Geometry: final body of the model. Coordinates: model frame, mm. A direction names the side the tool comes from. Give positions to 0.01 mm unless a question says otherwise; leave off trailing zeros. Loops run counter-clockwise (first coordinate to the right, second up) from the corner with the lowest first, then second, coordinate; pieces in that order, holes last. Notation, with made-up numbers: (-38, -5.5) -> (-18, -5.5) arc R13 cw to (-18, 15.5) -> close; hole circle Ø6 at (88, -38.5). An arc over 180 degrees is marked (long way). Answer in a Markdown table with one row per item. Add a question column.
1) Access query for faces 1 (the cylindrical face through (-113.36, 142.48, 6.34)), 2 (the flat face through (72.745, 132.247, 10.647)), 3 (the flat face through (80, 65, 6)). Directions: +Z, -Z, +X, -X, +Y, -Y. A direction counts if a zero-diameter tool reaches every point of the face in a straight line with its end or side. Return the directions, or none.
2) Draft query along Y for faces 4 (the cylindrical face through (84, 251, 16)), 5 (the flat face through (-74.9, 66.2, 17.6)), 6 (the conical face through (-74.64, 25.81, 17.57)). Return one class per face: +Y half, -Y half, draft (parallel to the pull), parting line (faces both ways), or undercut.
3) Section query B-B (z = 17.75). Give the number of separate pieces and of enclosed holes in the cut face, plus the area to 3 significant figures.
4) Line query: line 1 (X direction, y = 212.5, z = 3.5); line 2 (X direction, y = 254, z = 18); line 3 (X direction, y = 47.5, z = 1.75). Output: solid intervals per line, ascending. Write a range as from..to.
5) Section query A-A (y = 81). Return the cut outline in (x, z).
6) First-contact query: P1, Ø8, axis at x = -88, z = 14.5, coming from the -Y side; P2, Ø1.2, axis at y = 61, z = 5.5, coming from the +X side; P3, Ø1, axis at y = 140.5, z = 19.5, coming from the -X side. Flat tips, straight axial feed; report the tip coordinate or a pass-through.
```python
from build123d import *

# Parameters (mm, degrees)
RESSALTO_EXTRUS_O1_DEPTH = 22.5
CHANFRO1_SIZE            = 10
CORTE_EXTRUS_O1_REACH    = 305.531
ESBO_O3_W                = 1139.230904301
ESBO_O3_H                = 709.798033895
CORTE_EXTRUS_O5_DEPTH    = 1.5
ESBO_O5_R                = 3
CORTE_EXTRUS_O6_DEPTH    = 304.423796035
CORTE_EXTRUS_O8_DEPTH    = 10


with BuildPart() as part:
    # Esboço1 → Ressalto-extrusão1 (new, symmetric)
    with BuildSketch(Plane.XY):
        with BuildLine():
            Line((-55.336923418, 0), (55.336923418, 0))
            ThreePointArc((55.336923418, 0), (59.563106036, 0.93692213), (62.99736785, 3.572123903))
            Line((62.99736785, 3.572123903), (77.660444431, 21.046898098))
            ThreePointArc((77.660444431, 21.046898098), (79.396926208, 24.054572761), (80, 27.474774195))
            Line((80, 27.474774195), (80, 103.835071852))
            ThreePointArc((80, 103.835071852), (81.685949179, 111.43989715), (86.427876097, 117.619696626))
            Line((86.427876097, 117.619696626), (108.572123903, 136.200926793))
            ThreePointArc((108.572123903, 136.200926793), (113.314050821, 142.380726268), (115, 149.985551567))
            Line((115, 149.985551567), (115, 249.022509221))
            ThreePointArc((115, 249.022509221), (114.06307787, 253.248691838), (111.427876097, 256.682953652))
            Line((111.427876097, 256.682953652), (86.427876097, 277.660444431))
            ThreePointArc((86.427876097, 277.660444431), (83.420201433, 279.396926208), (80, 280))
            Line((80, 280), (-80, 280))
            ThreePointArc((-80, 280), (-83.420201433, 279.396926208), (-86.427876097, 277.660444431))
            Line((-86.427876097, 277.660444431), (-111.427876097, 256.682953652))
            ThreePointArc((-111.427876097, 256.682953652), (-114.06307787, 253.248691838), (-115, 249.022509221))
            Line((-115, 249.022509221), (-115, 149.985551567))
            ThreePointArc((-115, 149.985551567), (-113.314050821, 142.380726268), (-108.572123903, 136.200926793))
            Line((-108.572123903, 136.200926793), (-86.427876097, 117.619696626))
            ThreePointArc((-86.427876097, 117.619696626), (-81.685949179, 111.43989715), (-80, 103.835071852))
            Line((-80, 103.835071852), (-80, 27.474774195))
            ThreePointArc((-80, 27.474774195), (-79.396926208, 24.054572761), (-77.660444431, 21.046898098))
            Line((-77.660444431, 21.046898098), (-62.99736785, 3.572123903))
            ThreePointArc((-62.99736785, 3.572123903), (-59.563106036, 0.93692213), (-55.336923418, 0))
        make_face()
        Polygon((-90, 146.725210262), (-90, 236.228675506), (-61.670438633, 260), (61.670438633, 260), (90, 236.228675506), (90, 146.725210262), (55, 117.356723171), (55, 28.676328085), (47.719696304, 20), (-47.719696304, 20), (-55, 28.676328085), (-55, 117.356723171), align=None, mode=Mode.SUBTRACT)
    extrude(amount=RESSALTO_EXTRUS_O1_DEPTH, both=True)

    # Chanfro1
    chanfro1_edges = [part.edges().sort_by_distance(p)[0] for p in [
        (-70.32890614, 12.309511, 22.5),
        (-59.563106036, 0.93692213, 22.5),
        (0, 0, 22.5),
        (59.563106036, 0.93692213, 22.5),
        (70.32890614, 12.309511, 22.5),
        (79.396926208, 24.054572761, 22.5),
        (80, 65.654923023, 22.5),
        (81.685949179, 111.43989715, 22.5),
        (97.5, 126.910311709, 22.5),
        (113.314050821, 142.380726268, 22.5),
        (115, 199.504030394, 22.5),
        (114.06307787, 253.248691838, 22.5),
        (98.927876097, 267.171699041, 22.5),
        (98.927876097, 267.171699041, -22.5),
        (114.06307787, 253.248691838, -22.5),
        (115, 199.504030394, -22.5),
        (113.314050821, 142.380726268, -22.5),
        (97.5, 126.910311709, -22.5),
        (81.685949179, 111.43989715, -22.5),
        (80, 65.654923023, -22.5),
        (79.396926208, 24.054572761, -22.5),
        (70.32890614, 12.309511, -22.5),
        (59.563106036, 0.93692213, -22.5),
        (0, 0, -22.5),
        (-59.563106036, 0.93692213, -22.5),
        (-70.32890614, 12.309511, -22.5),
        (-79.396926208, 24.054572761, -22.5),
        (-80, 65.654923023, -22.5),
        (-81.685949179, 111.43989715, -22.5),
        (-97.5, 126.910311709, -22.5),
        (-113.314050821, 142.380726268, -22.5),
        (-115, 199.504030394, -22.5),
        (-114.06307787, 253.248691838, -22.5),
        (-98.927876097, 267.171699041, -22.5),
        (-83.420201433, 279.396926208, -22.5),
        (0, 280, -22.5),
        (83.420201433, 279.396926208, -22.5),
        (83.420201433, 279.396926208, 22.5),
        (0, 280, 22.5),
        (-83.420201433, 279.396926208, 22.5),
        (-98.927876097, 267.171699041, 22.5),
        (-114.06307787, 253.248691838, 22.5),
        (-115, 199.504030394, 22.5),
        (-113.314050821, 142.380726268, 22.5),
        (-97.5, 126.910311709, 22.5),
        (-81.685949179, 111.43989715, 22.5),
        (-80, 65.654923023, 22.5),
        (-79.396926208, 24.054572761, 22.5),
    ]]
    chamfer(chanfro1_edges, length=CHANFRO1_SIZE - 0.0001)  # a hair under: the kernel refuses the full size

    # Esboço3 → Corte-extrusão1 (cut, up to next)
    with BuildSketch(Plane.XY, mode=Mode.PRIVATE) as corte_extrus_o1_sk1:
        with Locations((-153.157436203, 152.53565808)):
            Rectangle(ESBO_O3_W, ESBO_O3_H)
    corte_extrus_o1_tool1 = extrude(corte_extrus_o1_sk1.sketch, amount=-CORTE_EXTRUS_O1_REACH, mode=Mode.PRIVATE) & part.part
    add(corte_extrus_o1_tool1.solids().sort_by_distance((-153.157436, 152.535658, 0))[0], mode=Mode.SUBTRACT)

    # Esboço4 → Corte-extrusão5 (cut)
    with BuildSketch(Plane.XY.offset(22.5)):
        Polygon((-69, 27.838744429), (-54.87061576, 11), (54.87061576, 11), (69, 27.838744429), (69, 117.355452403), (104, 146.723939495), (104, 248.556201562), (79.636029766, 269), (-79.636029766, 269), (-104, 248.556201562), (-104, 146.723939495), (-69, 117.355452403), align=None)
        Polygon((-90, 146.725210262), (-90, 236.228675506), (-61.670438633, 260), (61.670438633, 260), (90, 236.228675506), (90, 146.725210262), (55, 117.356723171), (55, 28.676328085), (47.719696304, 20), (-47.719696304, 20), (-55, 28.676328085), (-55, 117.356723171), align=None, mode=Mode.SUBTRACT)
    extrude(amount=-CORTE_EXTRUS_O5_DEPTH, mode=Mode.SUBTRACT)

    # Esboço5 → Corte-extrusão6 (cut, through all)
    with BuildSketch(Plane.XY.offset(21)):
        with Locations((-97, 244)):
            Circle(ESBO_O5_R)
        with Locations((-62, 60.396230411)):
            Circle(ESBO_O5_R)
        with Locations((-84, 254)):
            Circle(ESBO_O5_R)
        with Locations((-55, 21)):
            Circle(ESBO_O5_R)
        with Locations(Location((55, 21, 0), (0, 0, 180))):
            Circle(ESBO_O5_R)
        with Locations(Location((84, 254, 0), (0, 0, 180))):
            Circle(ESBO_O5_R)
        with Locations(Location((62, 60.396230411, 0), (0, 0, 180))):
            Circle(ESBO_O5_R)
        with Locations(Location((97, 244, 0), (0, 0, 180))):
            Circle(ESBO_O5_R)
    extrude(amount=-CORTE_EXTRUS_O6_DEPTH, mode=Mode.SUBTRACT)

    # Esboço7 → Corte-extrusão8 (cut)
    with BuildSketch(Plane(origin=(0, 0, 0), x_dir=(-1, 0, 0), z_dir=(0, 0, -1))):
        Polygon((83.862394336, 258.039108567), (80.43322654, 255.900384282), (80.570832205, 251.861275715), (84.137605664, 249.960891433), (87.56677346, 252.099615718), (87.429167795, 256.138724285), align=None)
        Polygon((-96.731346334, 248.032512683), (-100.357931592, 246.248917241), (-100.626585258, 242.216404558), (-97.268653666, 239.967487317), (-93.642068408, 241.751082759), (-93.373414742, 245.783595442), align=None)
        Polygon((-62, 64.437682295), (-65.5, 62.416956353), (-65.5, 58.375504468), (-62, 56.354778526), (-58.5, 58.375504468), (-58.5, 62.416956353), align=None)
        Polygon((-84, 258.041451884), (-87.5, 256.020725942), (-87.5, 251.979274058), (-84, 249.958548116), (-80.5, 251.979274058), (-80.5, 256.020725942), align=None)
        Polygon((54.761641425, 25.034416751), (51.386913316, 22.810783794), (51.625271892, 18.776367043), (55.238358575, 16.965583249), (58.613086684, 19.189216206), (58.374728108, 23.223632957), align=None)
        Polygon((62, 64.437682295), (58.5, 62.416956353), (58.5, 58.375504468), (62, 56.354778526), (65.5, 58.375504468), (65.5, 62.416956353), align=None)
        Polygon((97, 248.041451884), (93.5, 246.020725942), (93.5, 241.979274058), (97, 239.958548116), (100.5, 241.979274058), (100.5, 246.020725942), align=None)
        Polygon((-55.334155485, 25.027613865), (-58.655093666, 22.724419793), (-58.320938181, 18.696805928), (-54.665844515, 16.972386135), (-51.344906334, 19.275580207), (-51.679061819, 23.303194072), align=None)
    extrude(amount=-CORTE_EXTRUS_O8_DEPTH, mode=Mode.SUBTRACT)


solid = part.part
```
Evaluation:
| question | item | result |
|---|---|---|
| 1 | face 1 | +Z, -Z, -X, -Y |
| 1 | face 2 | +Z, -Z |
| 1 | face 3 | +Z, -Z, +X, -Y |
| 2 | face 4 | undercut |
| 2 | face 5 | draft |
| 2 | face 6 | -Y half |
| 3 | separate pieces | 1 |
| 3 | enclosed holes | 9 |
| 3 | area | 14,600 mm² |
| 4 | line 1 | -115..-90, 90..115 |
| 4 | line 2 | -106.07..-87, -81..-68.82, 68.82..81, 87..106.07 |
| 4 | line 3 | -80..-55, 55..80 |
| 5 | outline | (-80, 0) -> (-55, 0) -> (-55, 21) -> (-69, 21) -> (-69, 22.5) -> (-70, 22.5) -> (-80, 12.5) -> close; (55, 0) -> (80, 0) -> (80, 12.5) -> (70, 22.5) -> (69, 22.5) -> (69, 21) -> (55, 21) -> close |
| 6 | P1 | y = 115.78 |
| 6 | P2 | x = 80 |
| 6 | P3 | x = -103.79 |
